from build123d import *

# Parameters (mm, degrees)
F1_DEPTH = 50.8


with BuildPart() as f1:
    # F0 (on Front) → F1 (new body, symmetric)
    with BuildSketch(Plane.XZ):
        Polygon((6.35, 88.9), (0, 88.9), (0, 0), (133.35, 0), (133.35, 12.7), (6.35, 12.7), align=None)
    extrude(amount=F1_DEPTH, both=True)

    # F2 (on Front) → F3 (revolve, cut)
    with BuildSketch(Plane.XZ):
        Polygon((73.3769804781, 21.0355088013), (64.5556530526, -28.9927250518), (108.330357674, -36.711386549), (120.65, 12.7), align=None)
    revolve(axis=Axis((68.9663167654, 0, -3.9786081252), (0.1736481777, 0, 0.984807753)), mode=Mode.SUBTRACT)


solid = f1.part
Verification items for the finished model (mm, model axes). A direction names the side the tool comes from. Give positions to 0.01 mm unless a question says otherwise; leave off trailing zeros. Loops run counter-clockwise (first coordinate to the right, second up) from the corner with the lowest first, then second, coordinate; pieces in that order, holes last.
1. Cross-section at B-B on z = 30. Record the cut outline in (x, y).
Derived:
outline: (0, -50.8) - (6.35, -50.8) - (6.35, 50.8) - (0, 50.8) - close
2. Release check for a two-part mould opening along Y. For faces 1 (the conical face through (95.696, 39.609, 2.182)), 2 (the flat face through (3, -1, 88.9)), 3 (the flat face through (56, 50.8, 12)) record: +Y half, -Y half, draft (parallel to the pull), parting line (faces both ways), or undercut.
Derived:
face 1: undercut
face 2: draft
face 3: +Y half
3. Tool access check on faces 4 (the flat face through (6.35, -1, 50)), 5 (the flat face through (21, -1, 0)). Record the directions out of +Z, -Z, +X, -X, +Y, -Y that give a thin tool (end or side, any length) a straight path to the whole face; none if there is none.
Derived:
face 4: +Z, +X, +Y, -Y
face 5: -Z, +X, -X, +Y, -Y
4. Cross-section at A-A on x = 19.5. Record the cut outline in (y, z).
Derived:
outline: (-50.8, 0) - (50.8, 0) - (50.8, 12.7) - (-50.8, 12.7) - close
5. Material ranges on probe 1 along Z at (x, y) = (28.5, 42); probe 2 along X at (y, z) = (11.5, 67.5); probe 3 along Y at (x, z) = (111.5, 7), recorded low to high.
Derived:
probe 1: z = 0 to 12.7
probe 2: x = 0 to 6.35
probe 3: y = -50.8 to -25.64, 25.64 to 50.8
6. Go/stop test with a flat-tipped pin: P1, Ø10, axis at x = 96.5, z = 15, coming from the +Y side. Record where the tip stops, or that it passes through.
Derived:
P1: stops at y = 50.8
